For this review, take the finished solid that the model builds, in its own axes (mm). A direction names the side the tool comes from. Coordinates: 2 decimals unless noted, no trailing zeros. Order: outer loops, then holes, each group sorted by start corner. A loop starts at its lowest first (then second) coordinate and runs counter-clockwise, first axis right, second up. Notation, with made-up numbers: M 24,-31.5 L 47,-31.5 A15 ccw 47,-6.5 Z; hole C 24,83 d5. An arc over 180 degrees is marked long. Use CSV: the item, a comma, the result in double quotes.
```python
from build123d import *

# Parameters (mm, degrees)
F0_W     = 40
F0_H     = 40
F1_DEPTH = 10
F2_R     = 4
F3_DEPTH = 10.001
F4_W     = 1.5
F4_H     = 5
F5_DEPTH = 3
F6_W     = 13
F6_H     = 5
F7_DEPTH = 2


with BuildPart() as f1:
    # F0 (on Top) → F1 (new body)
    with BuildSketch(Plane.XY):
        with Locations((20, -20)):
            Rectangle(F0_W, F0_H)
    extrude(amount=F1_DEPTH)

    # F2 (on face) → F3 (cut, through all)
    with BuildSketch(Plane.XY.offset(10)):
        with Locations((20, -20)):
            Circle(F2_R)
    extrude(amount=-F3_DEPTH, mode=Mode.SUBTRACT)

    # F4 (on face) → F5 (join)
    with BuildSketch(Plane.YZ.offset(40)):
        with Locations((-25.75, 5)):
            Rectangle(F4_W, F4_H)
        with Locations((-14.25, 5)):
            Rectangle(F4_W, F4_H)
    extrude(amount=F5_DEPTH)

    # F6 (on face) → F7 (join)
    with BuildSketch(Plane.YZ.offset(43)):
        with Locations((-20, 5)):
            Rectangle(F6_W, F6_H)
    extrude(amount=F7_DEPTH)


solid = f1.part
```
Item 1: Add section B-B on z = 4.25. State the section outline as (x, y) points, and give its area (3 significant figures).
Solutions:
outline,"M 0,-40 L 40,-40 L 40,-26.5 L 45,-26.5 L 45,-13.5 L 40,-13.5 L 40,0 L 0,0 Z; hole C 20,-20 d8; hole M 40,-25 L 43,-25 L 43,-15 L 40,-15 Z"
area,"1,580 mm^2"
Item 2: Add section A-A on y = -15.5. State the section outline as (x, z) points.
Solutions:
outline,"M 0,0 L 40,0 L 40,10 L 0,10 Z; M 43,2.5 L 45,2.5 L 45,7.5 L 43,7.5 Z"
Item 3: Add section D-D on z = 1.75. State the section outline as (x, y) points, and give its area (3 significant figures).
Solutions:
outline,"M 0,-40 L 40,-40 L 40,0 L 0,0 Z; hole C 20,-20 d8"
area,"1,550 mm^2"
Item 4: Draft analysis for pull direction X (two halves, no side actions). For faces 1 (the face through (40, -20, 5)), 2 (the face through (45, -20, 5)), 3 (the face through (42, -13.5, 5)), state which applies: released by +X, released by -X, zero draft, split by the parting line, or undercut.
Solutions:
face 1,"undercut"
face 2,"released by +X"
face 3,"zero draft"
Item 5: Add section C-C on x = 20. State the section outline as (y, z) points, and give its area (3 significant figures).
Solutions:
outline,"M -40,0 L -24,0 L -24,10 L -40,10 Z; M -16,0 L 0,0 L 0,10 L -16,10 Z"
area,"320 mm^2"
Item 6: For faces 4 (the face through (42, -26.5, 5)), 5 (the face through (44, -20, 7.5)), 6 (the face through (41, -25, 5)), 7 (the face through (44, -20, 2.5)), list the 3-axis set-ups (+Z, -Z, +X, -X, +Y, -Y) from which the entire face can be reached by the end or side of a thin tool; tool diameter is ignored.
Solutions:
face 4,"+Z, -Z, +X, -Y"
face 5,"+Z, +X, +Y, -Y"
face 6,"+Z, -Z"
face 7,"-Z, +X, +Y, -Y"
Item 7: To check wall thickness, follow line 1 along Y through (x, z) = (20, 6); line 2 along X through (y, z) = (-22, 4.5); line 3 along X through (y, z) = (-27, 6.75). State the ranges of each line that lie inside material, in increasing order. Write a range as [from, to].
Solutions:
line 1,"[-40, -24], [-16, 0]"
line 2,"[0, 16.54], [23.46, 40], [43, 45]"
line 3,"[0, 40]"
Item 8: Clearance check with flat-ended pins moving along their axes: pin 1 Ø1 at (x, y) = (36, -8) entering from -Z; pin 2 Ø1.5 at (x, y) = (42.5, -20.5) entering from +Z; pin 3 Ø5.5 at (x, z) = (43.5, 5) entering from -Y; pin 4 Ø4 at (x, z) = (43.5, 4.5) entering from +Y. State where each tip first meets the part, or that it passes through.
Solutions:
pin 1,"z = 0"
pin 2,"z = 7.5"
pin 3,"y = -26.5"
pin 4,"y = -13.5"
